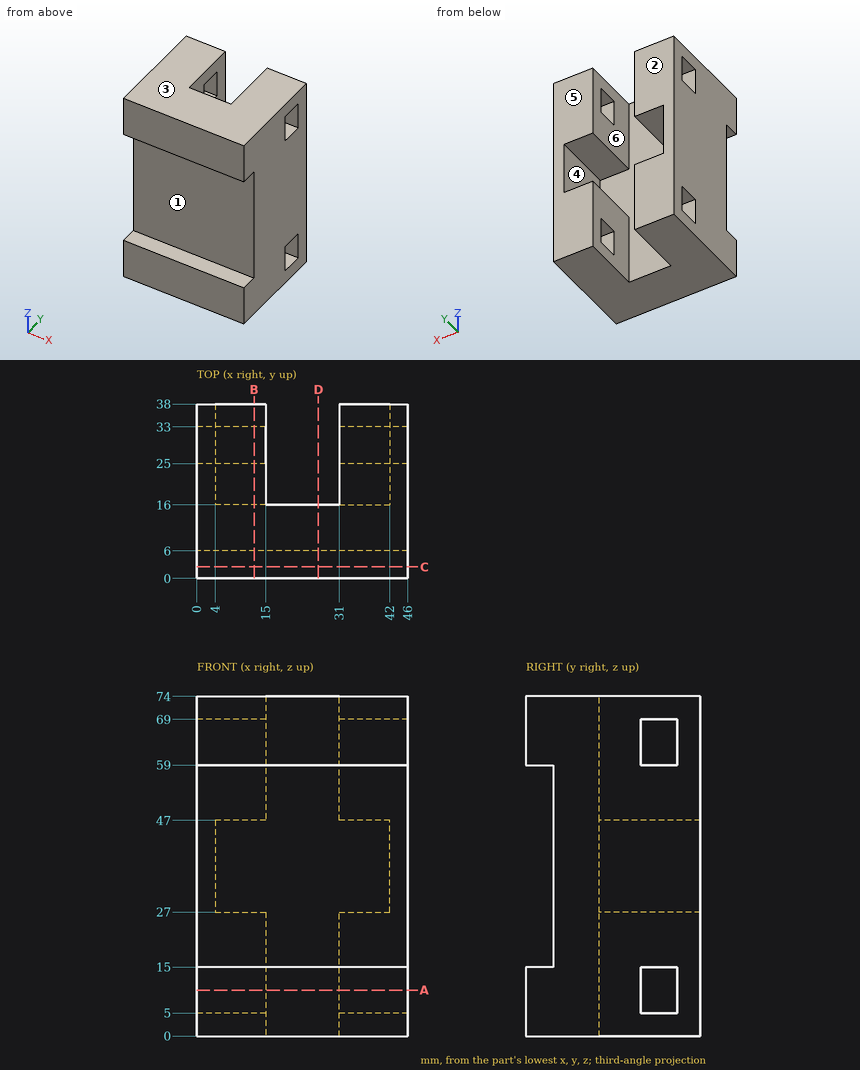
Here's the drawing with two shaded views (mm, measured from the low corner). I have some questions. A direction names the side the tool comes from. Give positions to 0.01 mm unless a question says otherwise; leave off trailing zeros. Loops run counter-clockwise (first coordinate to the right, second up) from the corner with the lowest first, then second, coordinate; pieces in that order, holes last. Notation, with made-up numbers: M -22.75,-16 L 8.25,-16 A18 ccw 8.25,11 Z; hole C 24,12.25 d2. An arc over 180 degrees is marked long. One line per item, written item: value.
(1) Suppose I cut it at C-C on y = 2.5. List the corners of the cut face in (x, z) for me, plus the area to 3 significant figures.
Returned:
outline: M 0,0 L 46,0 L 46,15 L 0,15 Z; M 0,59 L 46,59 L 46,74 L 0,74 Z
area: 1,380 mm^2
(2) I need wall thicknesses on line 1 (Z direction, x = 32.5, y = 25.5); line 2 (X direction, y = 35.5, z = 27.5); line 3 (Y direction, x = 4, z = 5.5). Which ranges of each line are inside material? Lowest first, please.
Returned:
line 1: 0 to 5, 15 to 27, 47 to 59, 69 to 74
line 2: 0 to 4, 42 to 46
line 3: 0 to 25, 33 to 38
(3) Will these pins go through, and if not, where does the flat tip stop? pin 1 (8 mm diameter, centred on x = 37.5, y = 23.5, fed in from -Z); pin 2 (6 mm diameter, centred on x = 12, z = 44, fed in from -Y); pin 3 (5 mm diameter, centred on x = 23, z = 65.5, fed in from +Y).
Returned:
pin 1: z = 0
pin 2: y = 6
pin 3: y = 16
(4) Suppose I cut it at D-D on x = 26.5. List the corners of the cut face in (y, z) for me, plus the area to 3 significant figures.
Returned:
outline: M 0,0 L 16,0 L 16,74 L 0,74 L 0,59 L 6,59 L 6,15 L 0,15 Z
area: 920 mm^2
(5) Suppose I cut it at A-A on z = 10. List the corners of the cut face in (x, y) for me.
Returned:
outline: M 0,0 L 46,0 L 46,25 L 31,25 L 31,16 L 15,16 L 15,25 L 0,25 Z; M 0,33 L 15,33 L 15,38 L 0,38 Z; M 31,33 L 46,33 L 46,38 L 31,38 Z
(6) Which directions (+Z, -Z, +X, -X, +Y, -Y) give clear straight access to the entire face, cutting with the end or side of a thin tool? Please do the marked faces 4, 5 and 6.
Returned:
face 4: +Y
face 5: +Z, -Z, +X, -X, +Y
face 6: +Z, -Z, +Y
(7) We'd pull the mould along Z, two halves only. Please class the marked faces 1, 2 and 3: released by +Z, released by -Z, zero draft, split by the parting line, or undercut.
Returned:
face 1: undercut
face 2: zero draft
face 3: released by +Z
(8) Suppose I cut it at B-B on x = 12.5. List the corners of the cut face in (y, z) for me.
Returned:
outline: M 0,0 L 38,0 L 38,27 L 16,27 L 16,47 L 38,47 L 38,74 L 0,74 L 0,59 L 6,59 L 6,15 L 0,15 Z; hole M 25,5 L 33,5 L 33,15 L 25,15 Z; hole M 25,59 L 33,59 L 33,69 L 25,69 Z
